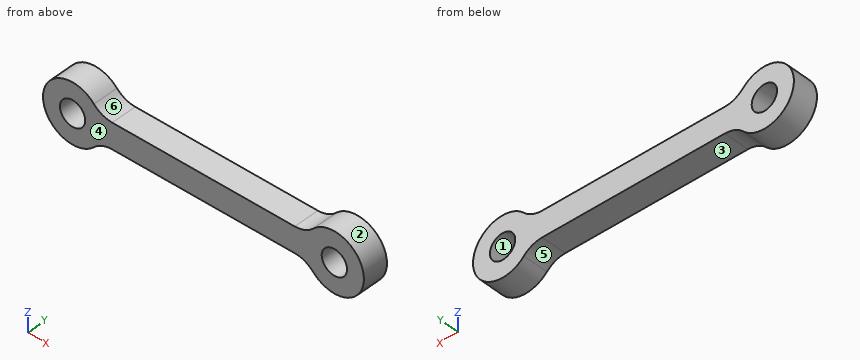
```python
from build123d import *

# Parameters (mm, degrees)
SKETCH1_R           = 1.5
BOSS_EXTRUDE1_DEPTH = 3
FILLET1_R           = 3


with BuildPart() as part:
    # Sketch1 → Boss-Extrude1 (new body)
    with BuildSketch(Plane(origin=(0, 0, 0), x_dir=(1, 0, 0), z_dir=(0, 1, 0))):
        with BuildLine():
            Line((-12.33772234, 1.5), (12.33772234, 1.5))
            ThreePointArc((12.33772234, 1.5), (19, 0), (12.33772234, -1.5))
            Line((12.33772234, -1.5), (-12.33772234, -1.5))
            ThreePointArc((-12.33772234, -1.5), (-19, 0), (-12.33772234, 1.5))
        make_face()
        with Locations((-15.5, 0)):
            Circle(SKETCH1_R, mode=Mode.SUBTRACT)
        with Locations((15.5, 0)):
            Circle(SKETCH1_R, mode=Mode.SUBTRACT)
    extrude(amount=BOSS_EXTRUDE1_DEPTH)

    # Fillet1
    fillet1_edges = [part.edges().sort_by_distance(p)[0] for p in [
        (-12.33772234, 1.5, -1.5),
        (12.33772234, 1.5, -1.5),
        (12.33772234, 1.5, 1.5),
        (-12.33772234, 1.5, 1.5),
    ]]
    fillet(fillet1_edges, radius=FILLET1_R)


solid = part.part
```
Check sheet for the modelled part. Datum: model origin and axes. Units: mm. Face numbers are marked on the shaded views. A direction names the side the tool comes from. Give positions to 0.01 mm unless a question says otherwise; leave off trailing zeros. Order: outer loops, then holes, each group sorted by start corner. A loop starts at its lowest first (then second) coordinate and runs counter-clockwise, first axis right, second up. Notation, with made-up numbers: M -20.75,-20 L -3.75,-20 A18 ccw -3.75,1 Z; hole C 58,2 d11. An arc over 180 degrees is marked long. Answer in a Markdown table with one row per item. Add a question column.
Q1. Sectioned sample at A-A, the plane z = 0. Record the boundary of the cut face in (x, y), and give its area (3 significant figures).
Q2. Thickness scan on L1, parallel to X at y = 2.3, z = 0; L2, parallel to Z at x = 15.5, y = 2.25; L3, parallel to X at y = 1.85, z = 0.5. Record the ranges inside material, lowest first.
Q3. Access from +Z, -Z, +X, -X, +Y, -Y to the whole of each face (thin tool, end or side, straight path). Record for the marked faces 4, 5 and 6.
Q4. Sectioned sample at D-D, the plane x = -1. Record the boundary of the cut face in (y, z), and give its area (3 significant figures).
Q5. Gauge pin test, flat ends, axial feed: pin 1 Ø2 at (x, z) = (14.5, 1.5) entering from -Y; pin 2 Ø2.5 at (x, z) = (15.5, 0) entering from +Y. Record the tip position at first contact, or that the pin passes through.
Q6. Release check for a two-part mould opening along Z. For the marked faces 1, 2 and 3 record: released by +Z, released by -Z, zero draft, split by the parting line, or undercut.
Q7. Sectioned sample at B-B, the plane x = -15.5. Record the boundary of the cut face in (y, z).
Q8. Sectioned sample at C-C, the plane y = 1.05. Record the boundary of the cut face in (x, z).
Verdict:
| question | item | result |
|---|---|---|
| 1 | outline | M -19,0 L -17,0 L -17,3 L -19,3 Z; M -14,0 L 14,0 L 14,3 L -14,3 Z; M 17,0 L 19,0 L 19,3 L 17,3 Z |
| 1 | area | 96.0 mm² |
| 2 | L1 | -19 to -17, -14 to 14, 17 to 19 |
| 2 | L2 | -3.5 to -1.5, 1.5 to 3.5 |
| 2 | L3 | -18.96 to -16.91, -14.09 to 14.09, 16.91 to 18.96 |
| 3 | face 4 | +Z, -Z, +X, -X, -Y |
| 3 | face 5 | -Z, +Y, -Y |
| 3 | face 6 | +Z, +Y, -Y |
| 4 | outline | M 0,-1.5 L 3,-1.5 L 3,1.5 L 0,1.5 Z |
| 4 | area | 9.00 mm² |
| 5 | pin 1 | y = 0 |
| 5 | pin 2 | through |
| 6 | face 1 | undercut |
| 6 | face 2 | split by the parting line |
| 6 | face 3 | released by -Z |
| 7 | outline | M 0,-3.5 L 3,-3.5 L 3,-1.5 L 0,-1.5 Z; M 0,1.5 L 3,1.5 L 3,3.5 L 0,3.5 Z |
| 8 | outline | M -12.97,-2.42 A3 cw -10.81,-1.5 L 10.81,-1.5 A3 cw 12.97,-2.42 A3.5 ccw long 12.97,2.42 A3 cw 10.81,1.5 L -10.81,1.5 A3 cw -12.97,2.42 A3.5 ccw long Z; hole C -15.5,0 d3; hole C 15.5,0 d3 |
